Autodesk Inventor part; units mm, degrees
ref_plane "YZ Plane" through (0, 0, 0) normal (1, 0, 0) x (0, 1, 0)
ref_plane "XZ Plane" through (0, 0, 0) normal (0, 1, 0) x (-1, 0, 0)
ref_plane "XY Plane" through (0, 0, 0) normal (0, 0, 1) x (1, 0, 0)
sketch "Sketch1" plane through (0, 0, 0) normal (0, 0, 1) x (1, 0, 0)
  circle A0 centre (0, 0) radius 2.413
  dimension "d0" = 4.826
extrude "Extrusion1" add sketch "Sketch1" along normal blind 15.875
sketch "Sketch2" plane through (0, 0, 0) normal (0, 1, 0) x (-1, 0, 0)
  line L0 (0, 0) -> (0, -2.5654)
  line L1 (0, 0) -> (4.3239, 0)
  line L2 (0, -2.5654) -> (2.032, -2.5654)
  line L3 (4.3239, 0) -> (4.3239, 3.8864) construction
  arc A0 (4.5568, -0.3781) -> (4.3239, 0) centre (4.3239, -0.2608) ccw
  arc A1 (2.032, -2.5654) -> (4.5568, -0.3781) centre (0.6382, 1.5944) ccw
  line L4 (4.5847, 0.6553) -> (4.5847, -0.2608) construction
  dimension "d3" = 2.5654
  dimension "d6" = 2.032
  dimension "d12" = 4.5847
revolve "Revolution1" add sketch "Sketch2" angle 360 about axis through (0, 0, 0) along (0, 0, -1)
sketch "Sketch3" plane through (0, 0, -2.5654) normal (0, 0, -1) x (-1, 0, 0)
  circle A0 centre (0, 0) radius 2.032
  line L0 (-0.9165, 1.5875) -> (0.9165, 1.5875)
  line L1 (0.9165, 1.5875) -> (1.8331, 0)
  line L2 (1.8331, 0) -> (0.9165, -1.5875)
  line L3 (0.9165, -1.5875) -> (-0.9165, -1.5875)
  line L4 (-0.9165, -1.5875) -> (-1.8331, 0)
  line L5 (-1.8331, 0) -> (-0.9165, 1.5875)
  dimension "d8" = 3.175
extrude "Extrusion2" cut sketch "Sketch3" against normal blind 1.5875 contours L0 L1 L2 L3 L4 L5
chamfer "Chamfer1" distance 0.508 angle 45 1 edges at (-2.413, 0, 15.875)
thread "Thread1"
properties part number "10-32 x625 button head" material "Steel"
Model file for the job. Use its own axes, mm. A direction names the side the tool comes from. Round coordinates to 2 decimals unless told otherwise and drop trailing zeros. Write each loop counter-clockwise with the first axis right and the second up, starting at its lowest first coordinate (ties: lowest second). Pieces come first, ordered by that corner, then holes. Notation, with made-up numbers: (74.5, 24) - (121.5, 24) arc R16 ccw to (121.5, 28) - close; hole circle Ø1 at (-19, -9.75). An arc over 180 degrees is marked (long way). Use CSV: the item, a comma, the result in double quotes. Start each with the question number.
Item 1: Two-plate mould, pull along Y, no slides. Class faces 1 (the face through (0, 0, 15.875)), 2 (the face through (-1.37, 0.8, -1.78)), 3 (the face through (-1.915, 1.468, 7.576)): released by +Y, released by -Y, zero draft, split by the parting line, or undercut.
Item 2: Drill centre lines: L1, parallel to Z at x = -1, y = -0.75 (3 decimals); L2, parallel to Y at x = -0.25, z = 5.25; L3, parallel to Y at x = 2, z = 11.25. Where is each one in solid material? Low to high. Write a range as [from, to].
Item 3: Band-saw the part on A-A (z = 7.75). Write the cut outline in (x, y), and give its area (3 significant figures).
Item 4: Tool access for faces 4 (the face through (-1.381, -0.783, -1.783)), 5 (the face through (-2, -2, 0)): list every direction of +Z, -Z, +X, -X, +Y, -Y with a clear straight run to the whole face (end or side of a thin tool).
Item 5: Pin check, flat tips, straight feed: P1, Ø2, axis at x = -2, y = 3.5, coming from the +Z side; P2, Ø2, axis at x = 3, y = 0.5, coming from the +Z side; P3, Ø1.6, axis at x = 0, y = 0.5, coming from the -Z side. Stop position of each tip, or through.
Checked values:
1,face 1,"zero draft"
1,face 2,"undercut"
1,face 3,"split by the parting line"
2,L1,"z = [-0.978, 15.875]"
2,L2,"y = [-2.4, 2.4]"
2,L3,"y = [-1.35, 1.35]"
3,outline,"circle Ø4.83 at (0, 0)"
3,area,"18.3 mm²"
4,face 4,"-Z"
4,face 5,"+Z"
5,P1,"stops at z = 0"
5,P2,"stops at z = 15.74"
5,P3,"stops at z = -0.98"
